Model file for the job. Use its own axes, mm. A direction names the side the tool comes from. Round coordinates to 2 decimals unless told otherwise and drop trailing zeros. Loops run counter-clockwise (first coordinate to the right, second up) from the corner with the lowest first, then second, coordinate; pieces in that order, holes last. Notation, with made-up numbers: M 75.5,10 L 105.5,10 A26 ccw 105.5,37 Z; hole C 43.5,-30 d8. An arc over 180 degrees is marked long. Use a Markdown table: item, result. Add a question column.
Item 1: Wall check: L1, parallel to X at y = 4, z = 1.75; L2, parallel to Y at x = -1, z = -2.5; L3, parallel to Z at x = 15.5, y = 1. Give the ranges that are in metal, low to high. Write a range as from..to.
Item 2: Saw through at A-A on y = -4. Write the cut outline in (x, z), then the cut area to 3 significant figures.
Item 3: Two-plate mould, pull along X, no slides. Class faces 3 (the cylindrical face through (19.07, -1.38, -3.35)), 4 (the flat face through (0, 1, -4.762)), 5 (the flat face through (-10.478, -4, 0)): +X half, -X half, draft (parallel to the pull), parting line (faces both ways), or undercut.
Item 4: Saw through at B-B on y = 3.5. Write the cut outline in (x, z), then the cut area to 3 significant figures.
Item 5: Saw through at D-D on x = 1.5. Write the cut outline in (y, z).
Item 6: Pin check, flat tips, straight feed: P1, Ø3, axis at x = 0, z = -1.5, coming from the -Y side; P2, Ø2.5, axis at y = -5, z = 2, coming from the -X side. Stop position of each tip, or through.
Item 7: Saw through at C-C on z = 4.25. Write the cut outline in (x, y), then the cut area to 3 significant figures.
Item 8: Tool access for faces 1 (the flat face through (10.478, -4, 0)), 2 (the cylindrical face through (19, -1.38, 3.42)): list every direction of +Z, -Z, +X, -X, +Y, -Y with a clear straight run to the whole face (end or side of a thin tool).
```python
from build123d import *

# Parameters (mm, degrees)
SKETCH1_W                       = 41.275
SKETCH1_H                       = 9.525
BOSS_EXTRUDE1_DEPTH             = 6.35
SKETCH2_W                       = 10.16
SKETCH2_H                       = 9.525
BOSS_EXTRUDE2_DEPTH             = 8.89
F_7_32_0_21875_DIAMETER_HOLE1_D = 5.55625
FILLET1_R                       = 5.08


with BuildPart() as part:
    # Sketch1 → Boss-Extrude1 (new body)
    with BuildSketch(Plane(origin=(0, 0, 0), x_dir=(1, 0, 0), z_dir=(0, 1, 0))):
        Rectangle(SKETCH1_W, SKETCH1_H)
    extrude(amount=BOSS_EXTRUDE1_DEPTH)

    # Sketch2 → Boss-Extrude2 (add)
    with BuildSketch(Plane.XZ):
        with Locations((-15.5575, 0)):
            Rectangle(SKETCH2_W, SKETCH2_H)
        with Locations((15.5575, 0)):
            Rectangle(SKETCH2_W, SKETCH2_H)
    extrude(amount=BOSS_EXTRUDE2_DEPTH)

    # 7/32 (0.21875) Diameter Hole1 (through all)
    with Locations(Plane(origin=(0, 6.35, 0), x_dir=(1, 0, 0), z_dir=(0, 1, 0))):
        with Locations((-15.8115, 0), (15.9385, 0)):
            Hole(F_7_32_0_21875_DIAMETER_HOLE1_D / 2)

    # Fillet1
    # the kernel refuses this fillet: 5.08 mm, written as the material it takes off along each edge
    with BuildSketch(Plane(origin=(20.6375, -21.59, -4.7625), x_dir=(0, 0, 1), z_dir=(0, 1, 0)), Plane(origin=(20.6375, -21.59, 4.7625), x_dir=(-1, 0, 0), z_dir=(0, 1, 0)), Plane(origin=(-20.6375, 19.05, -4.7625), x_dir=(0, 0, 1), z_dir=(0, -1, 0)), Plane(origin=(-20.6375, 19.05, 4.7625), x_dir=(1, 0, 0), z_dir=(0, -1, 0))) as fillet1_piece_1:
        with BuildLine():
            CenterArc((FILLET1_R, -FILLET1_R), FILLET1_R, 90, 90)
            Line((0, -FILLET1_R), (0, 0))
            Line((0, 0), (FILLET1_R, 0))
        make_face()
    extrude(amount=40.64, mode=Mode.SUBTRACT)


solid = part.part
```
Entries:
| question | item | result |
|---|---|---|
| 1 | L1 | -20.2..-17.97, -13.65..13.78, 18.1..20.2 |
| 1 | L2 | 0..6.35 |
| 1 | L3 | -4.76..-2.74, 2.74..4.76 |
| 2 | outline | M -20.63,0 A5.08 ccw -15.56,-4.76 L -10.48,-4.76 L -10.48,4.76 L -15.56,4.76 A5.08 ccw Z; M 10.48,-4.76 L 15.56,-4.76 A5.08 ccw 20.63,0 A5.08 ccw 15.56,4.76 L 10.48,4.76 Z; hole C -15.81,0 d5.56; hole C 15.94,0 d5.56 |
| 2 | area | 123 mm2 |
| 3 | face 3 | +X half |
| 3 | face 4 | draft |
| 3 | face 5 | undercut |
| 4 | outline | M -20.63,0 A5.08 ccw -15.56,-4.76 L 15.56,-4.76 A5.08 ccw 20.63,0 A5.08 ccw 15.56,4.76 L -15.56,4.76 A5.08 ccw Z; hole C -15.81,0 d5.56; hole C 15.94,0 d5.56 |
| 4 | area | 323 mm2 |
| 5 | outline | M 0,-4.76 L 6.35,-4.76 L 6.35,4.76 L 0,4.76 Z |
| 6 | P1 | y = 0 |
| 6 | P2 | x = -20.52 |
| 7 | outline | M -17.78,-8.89 L -10.48,-8.89 L -10.48,0 L 10.48,0 L 10.48,-8.89 L 17.78,-8.89 L 17.78,6.35 L -17.78,6.35 Z |
| 7 | area | 356 mm2 |
| 8 | face 1 | +Z, -Z, -Y |
| 8 | face 2 | +Z, +X, +Y, -Y |
